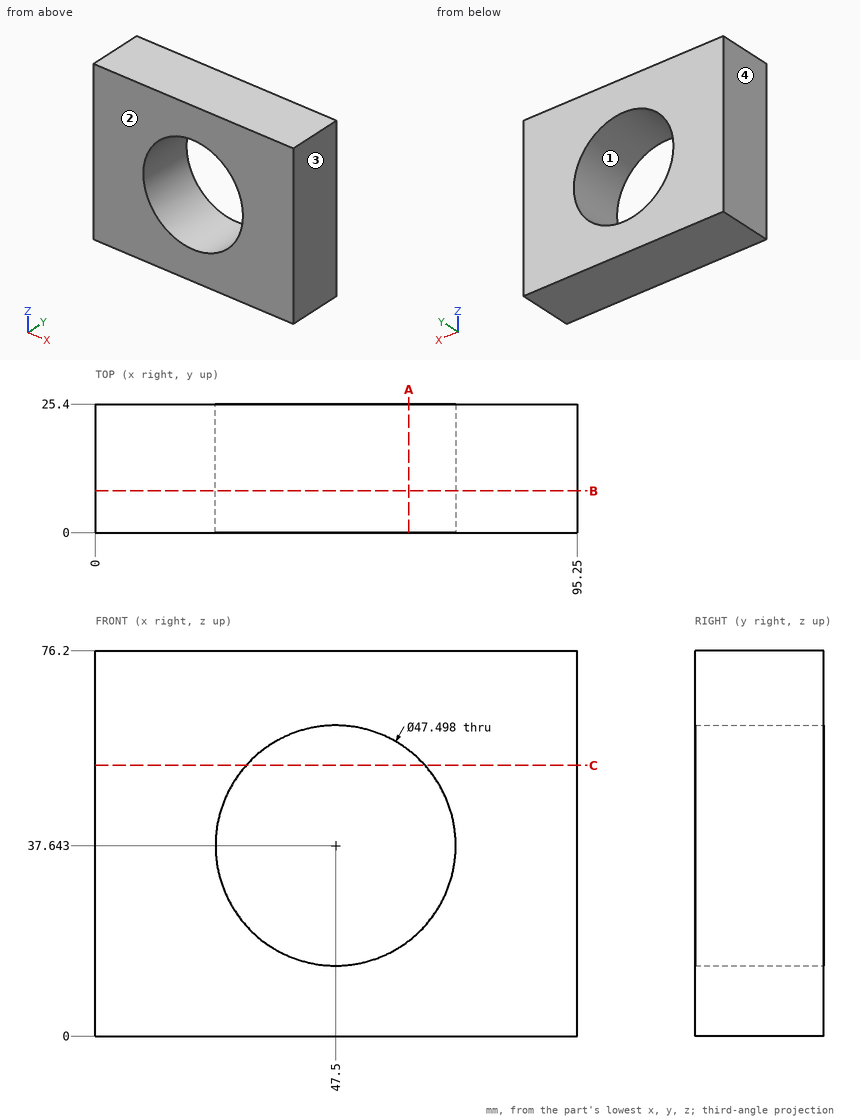
Design review of the part shown in the three views and the two pictorial views. Dimensions are in mm from the part's minimum x, y and z. Round coordinates to 2 decimals unless told otherwise and drop trailing zeros. Loops run counter-clockwise (first coordinate to the right, second up) from the corner with the lowest first, then second, coordinate; pieces in that order, holes last. Notation, with made-up numbers: (65, 24.5) - (95, 24.5) arc R21 cw to (95, 62.5) - close; hole circle Ø4 at (-6, 58). An arc over 180 degrees is marked (long way). Use one line per item in the form item = value.
1) We need section C-C on z = 53.5. Write out the cut boundary in (x, y).
Solutions:
outline = (0, 0) - (29.82, 0) - (29.82, 25.4) - (0, 25.4) - close; (65.18, 0) - (95.25, 0) - (95.25, 25.4) - (65.18, 25.4) - close
2) We need section B-B on y = 8.25. Write out the cut boundary in (x, z), then the cut area to 3 significant figures.
Solutions:
outline = (0, 0) - (95.25, 0) - (95.25, 76.2) - (0, 76.2) - close; hole circle Ø47.5 at (47.5, 37.64)
area = 5,490 mm2
3) Mouldability with a two-part tool opening along X and no side actions: class the marked faces 1, 2, 3 and 4 as pulls with the +X half, pulls with the -X half, needs draft (parallel to the pull), parting line crosses it, or undercut.
Solutions:
face_1 = undercut
face_2 = needs draft
face_3 = pulls with the +X half
face_4 = pulls with the -X half
4) We need section A-A on x = 62. Write out the cut boundary in (y, z) (1 decimal).
Solutions:
outline = (0, 0) - (25.4, 0) - (25.4, 18.8) - (0, 18.8) - close; (0, 56.5) - (25.4, 56.5) - (25.4, 76.2) - (0, 76.2) - close
5) Wall thickness on probe 1 along X at (y, z) = (18.25, 38.5); probe 2 along Z at (x, y) = (46.5, 19.25) (1 decimal); probe 3 along Z at (x, y) = (60, 21.5): over which ranges is each line inside the solid? List them lowest first.
Solutions:
probe_1 = 0 to 23.77, 71.23 to 95.25
probe_2 = 0 to 13.9, 61.4 to 76.2
probe_3 = 0 to 17.45, 57.84 to 76.2
